Input: part model. Units: mm. Frame: model coordinates. A direction names the side the tool comes from. Coordinates: 2 decimals unless noted, no trailing zeros. Write each loop counter-clockwise with the first axis right and the second up, starting at its lowest first coordinate (ties: lowest second). Pieces come first, ordered by that corner, then holes.
1) Line query: L1, parallel to Z at x = 1.75, y = 9; L2, parallel to Y at x = -6.25, z = -6.75; L3, parallel to X at y = -23.5, z = -6.25. Output: solid intervals per line, ascending.
2) Pin query (flat end, axial travel): pin 1 Ø1.6 at (y, z) = (-8.5, -1) entering from -X; pin 2 Ø2 at (x, z) = (1, -1.5) entering from -Y; pin 3 Ø4 at (x, z) = (2, -6.5) entering from +Y; pin 4 Ø12 at (x, y) = (-9, 18.5) entering from +Z. Return the tip coordinate at first contact, or that it passes through.
3) Section query D-D (y = -11.5). Output: boundary loops of the cut face in (x, z).
4) Section query A-A (x = 4.25). Output: boundary loops of the cut face in (y, z).
5) Draft query along X for faces 1 (the flat face through (0, -33, -8)), 2 (the flat face through (-9, -3, -5)), 3 (the flat face through (-11, -4, -8)). Return one class per face: pulls with the +X half, pulls with the -X half, needs draft (parallel to the pull), parting line crosses it, or undercut.
6) Set-up query: faces 4 (the flat face through (0, -31, -5)), 5 (the flat face through (9, 5, -5)), 6 (the flat face through (6, -25, -10)), 7 (the flat face through (10, -23, -7)). Return all of +Z, -Z, +X, -X, +Y, -Y with unobstructed straight access to the full face (end or side cutting, diameter ignored); none if empty.
7) Section query B-B (y = 5). Output: boundary loops of the cut face in (x, z).
8) Section query C-C (z = -7.75). Output: boundary loops of the cut face in (x, y), then the cut area to 3 significant figures.
from build123d import *

# Parameters (mm, degrees)
F1_DEPTH    = 11
F2_T        = -2
F3_DEPTH    = 25
F4_DEPTH    = 2
F5_DEPTH    = 2
F6_DEPTH    = 1
F7_T1_DEPTH = 65
F7_T3_DEPTH = 47
F7_T5_DEPTH = 83
F7_T7_DEPTH = 35


# Not quite as in the source:
# - a fillet or chamfer that OpenCascade refuses, or shapes differently, is made with other operations: its cross-section is extruded or revolved along the edge and cut away or added


with BuildPart() as f1:
    # F0 (on Top) → F1 (new body)
    with BuildSketch(Plane.XY):
        Polygon((11, -15), (11, 25), (-11, 25), (-11, -33), (11, -33), (11, -23), (6, -23), (6, -28), (-6, -28), (-6, -15), (-6, -5), (6, -5), (6, -15), align=None)
    extrude(amount=-F1_DEPTH)

    # F2
    f2_openings = [f1.faces().sort_by_distance(p)[0] for p in [
        (0, 25, -5.5),
    ]]
    offset(amount=F2_T, openings=f2_openings, kind=Kind.INTERSECTION)

    # F3 (cut): a face of the model
    f3_faces = [f1.faces().sort_by_distance(p)[0] for p in [
        (0, -3, -5.5),
    ]]
    extrude(f3_faces, amount=-F3_DEPTH, mode=Mode.SUBTRACT)

    # F4 (add): a face of the model
    f4_faces = [f1.faces().sort_by_distance(p)[0] for p in [
        (8, -14, -5.5),
    ]]
    extrude(f4_faces, amount=-F4_DEPTH)

    # F5 (add): a face of the model
    f5_faces = [f1.faces().sort_by_distance(p)[0] for p in [
        (8, -14, -5.5),
    ]]
    extrude(f5_faces, amount=-F5_DEPTH)

    # F6 (cut): faces of the model
    f6_faces = [f1.faces().sort_by_distance(p)[0] for p in [
        (8, -14, -5.5),
        (8, -24, -5.5),
    ]]
    extrude(f6_faces, amount=-F6_DEPTH, mode=Mode.SUBTRACT)

    # F7: fillet of radius 5 on 5 edges, made by hand

    # F7_s2 → F7_t1 (cut)
    with BuildSketch(Plane.XZ.offset(-37.5)):
        with BuildLine():
            ThreePointArc((11, -5), (9.5355339059, -1.4644660941), (6, 0))
            Line((6, 0), (11, 0))
            Line((11, 0), (11, -5))
        make_face()
    extrude(amount=F7_T1_DEPTH, mode=Mode.SUBTRACT)

    # F7_s4 → F7_t3 (cut)
    with BuildSketch(Plane.YZ.offset(-23.5)):
        with BuildLine():
            ThreePointArc((20, 0), (23.5355339059, -1.4644660941), (25, -5))
            Line((25, -5), (25, 0))
            Line((25, 0), (20, 0))
        make_face()
        with BuildLine():
            ThreePointArc((-33, -5), (-31.5355339059, -1.4644660941), (-28, 0))
            Line((-28, 0), (-33, 0))
            Line((-33, 0), (-33, -5))
        make_face()
    extrude(amount=F7_T3_DEPTH, mode=Mode.SUBTRACT)

    # F7_s6 → F7_t5 (cut)
    with BuildSketch(Plane.XZ.offset(-37.5)):
        with BuildLine():
            ThreePointArc((-11, -5), (-9.5355339059, -1.4644660941), (-6, 0))
            Line((-6, 0), (-11, 0))
            Line((-11, 0), (-11, -5))
        make_face()
    extrude(amount=F7_T5_DEPTH, mode=Mode.SUBTRACT)

    # F7_s8 → F7_t7 (cut)
    with BuildSketch(Plane.XZ.offset(10.5)):
        with BuildLine():
            ThreePointArc((11, -5), (9.5355339059, -1.4644660941), (6, 0))
            Line((6, 0), (11, 0))
            Line((11, 0), (11, -5))
        make_face()
    extrude(amount=F7_T7_DEPTH, mode=Mode.SUBTRACT)


solid = f1.part
Answer:
1. L1: z = -11 to -9, -2 to 0
1. L2: y = -33 to -31, -30 to -28
1. L3: x = -11 to -9, 9 to 11
2. pin 1: stops at x = -9.84
2. pin 2: stops at y = -32.33
2. pin 3: stops at y = -28
2. pin 4: stops at z = 0
3. outline: (-11, -11) - (-6, -11) - (-6, -9) - (-9, -9) - (-9, -2) - (-6, -2) - (-6, 0) arc R5 ccw to (-11, -5) - close; (6, -11) - (11, -11) - (11, -5) arc R5 ccw to (6, 0) - (6, -2) - (9, -2) - (9, -9) - (6, -9) - close
4. outline: (-33, -11) - (-28, -11) - (-28, 0) arc R5 ccw to (-33, -5) - close; (-5, -11) - (25, -11) - (25, -9) - (-5, -9) - close; (-5, -2) - (24, -2) arc R5 ccw to (20, 0) - (-5, 0) - close; hole (-31, -9) - (-30, -9) - (-30, -2) - (-31, -2) - close
5. face 1: needs draft
5. face 2: undercut
5. face 3: pulls with the -X half
6. face 4: none
6. face 5: +Y
6. face 6: +Z, -Z
6. face 7: +Z, -Z, +X
7. outline: (-11, -11) - (11, -11) - (11, -5) arc R5 ccw to (6, 0) - (-6, 0) arc R5 ccw to (-11, -5) - close; hole (-9, -9) - (9, -9) - (9, -2) - (-9, -2) - close
8. outline: (-11, -33) - (11, -33) - (11, -23) - (9, -23) - (9, -31) - (-9, -31) - (-9, 25) - (-11, 25) - close; (-8, -30) - (8, -30) - (8, -28) - (-8, -28) - close; (9, -15) - (11, -15) - (11, 25) - (9, 25) - close
8. area: 284 mm2
